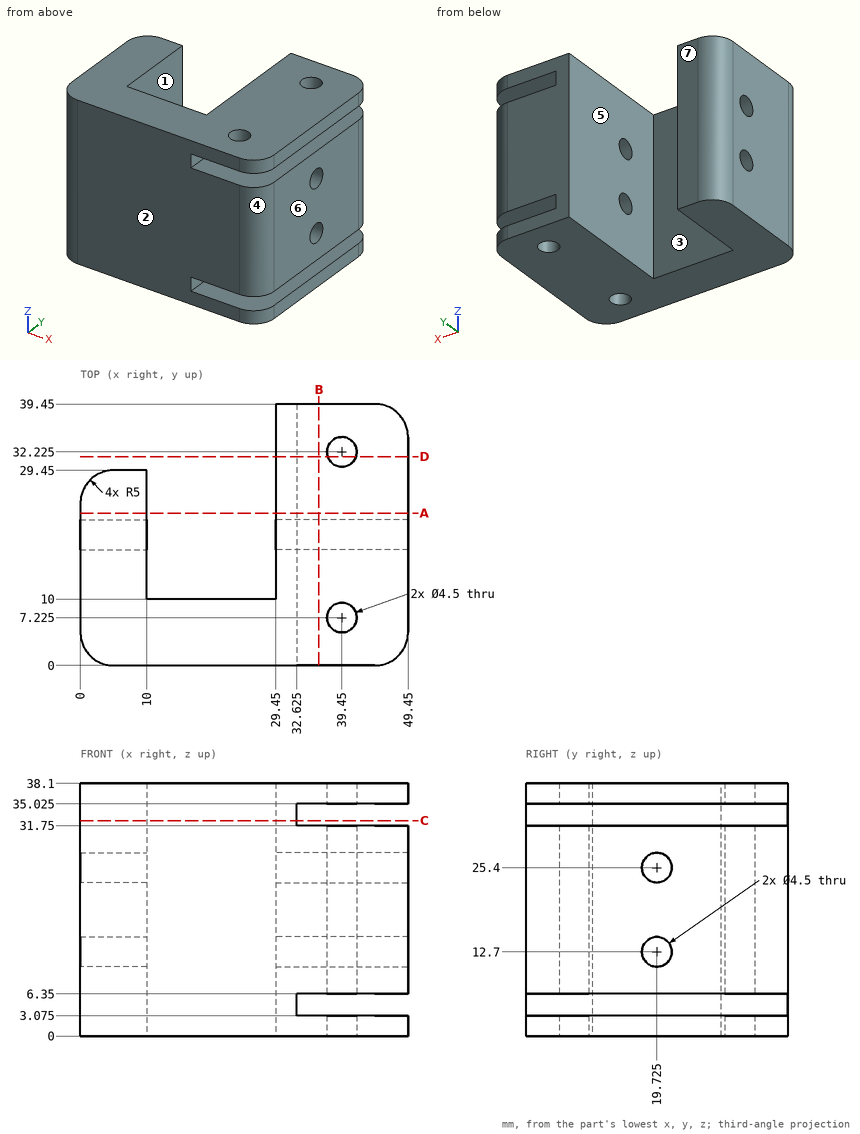
Geometry: see drawing. Coordinates: mm, zero at the bounding-box minimum. A direction names the side the tool comes from. Give positions to 0.01 mm unless a question says otherwise; leave off trailing zeros. Loops run counter-clockwise (first coordinate to the right, second up) from the corner with the lowest first, then second, coordinate; pieces in that order, holes last. Notation, with made-up numbers: (5, -10.5) - (38, -10.5) arc R9 ccw to (38, 3.5) - close; hole circle Ø10 at (-33.75, 57). An arc over 180 degrees is marked (long way). Use CSV: the item, a comma, the result in double quotes. Start each with the question number.
Item 1: Mould query, pull axis X, two halves, no side actions, for the marked faces 1, 2, 3 and 4. Classes: pulls with the +X half, pulls with the -X half, needs draft (parallel to the pull), parting line crosses it, or undercut.
Item 2: Section A-A on y = 23. Return loops of the section in (x, z) (3 decimals), then the cut area to 3 significant figures.
Item 3: Line query: line 1 (Y direction, x = 39.45, z = 36.7) (3 decimals); line 2 (Z direction, x = 45.5, y = 12) (3 decimals); line 3 (Y direction, x = 40.75, z = 12.7) (3 decimals). Output: solid intervals per line, ascending.
Item 4: Reachability of the marked faces 5, 6 and 7 from +Z, -Z, +X, -X, +Y, -Y: full face, straight path, thin tool, end or side. Return the list, or none.
Item 5: Section B-B on x = 36. Return loops of the section in (y, z) (3 decimals), then the cut area to 3 significant figures.
Item 6: Section D-D on y = 31.5. Return loops of the section in (x, z) (3 decimals).
Item 7: Section C-C on z = 32.5. Return loops of the section in (x, y) (3 decimals), then the cut area to 3 significant figures.
Item 8: Contact query for flat-ended pins moving along their axis: P1, Ø3, axis at x = 20, y = 12, coming from the -Z side; P2, Ø6, axis at x = 39.45, y = 32.225, coming from the +Z side; P3, Ø21.5, axis at x = 16, z = 12.5, coming from the +Y side. Output: stop coordinate, or through.
Ans:
1,face 1,"undercut"
1,face 2,"needs draft"
1,face 3,"undercut"
1,face 4,"pulls with the +X half"
2,outline,"(0, 0) - (10, 0) - (10, 38.1) - (0, 38.1) - close; (29.45, 0) - (49.45, 0) - (49.45, 3.075) - (32.625, 3.075) - (32.625, 6.35) - (49.45, 6.35) - (49.45, 31.75) - (32.625, 31.75) - (32.625, 35.025) - (49.45, 35.025) - (49.45, 38.1) - (29.45, 38.1) - close"
2,area,"1,030 mm2"
3,line 1,"y = 0 to 4.975, 9.475 to 29.975, 34.475 to 39.45"
3,line 2,"z = 0 to 3.075, 6.35 to 31.75, 35.025 to 38.1"
3,line 3,"y = 0 to 5.389, 9.061 to 17.475, 21.975 to 30.389, 34.061 to 39.45"
4,face 5,"+Z, -Z, +Y"
4,face 6,"+Z, -Z, +X, +Y, -Y"
4,face 7,"+Z, -Z, -X, +Y"
5,outline,"(0, 0) - (39.45, 0) - (39.45, 3.075) - (0, 3.075) - close; (0, 6.35) - (39.45, 6.35) - (39.45, 31.75) - (0, 31.75) - close; (0, 35.025) - (39.45, 35.025) - (39.45, 38.1) - (0, 38.1) - close; hole circle Ø4.5 at (19.725, 12.7); hole circle Ø4.5 at (19.725, 25.4)"
5,area,"1,210 mm2"
6,outline,"(29.45, 0) - (37.32, 0) - (37.32, 3.075) - (32.625, 3.075) - (32.625, 6.35) - (37.32, 6.35) - (37.32, 31.75) - (32.625, 31.75) - (32.625, 35.025) - (37.32, 35.025) - (37.32, 38.1) - (29.45, 38.1) - close; (41.58, 0) - (49.45, 0) - (49.45, 3.075) - (41.58, 3.075) - close; (41.58, 6.35) - (49.45, 6.35) - (49.45, 31.75) - (41.58, 31.75) - close; (41.58, 35.025) - (49.45, 35.025) - (49.45, 38.1) - (41.58, 38.1) - close"
7,outline,"(0, 5) arc R5 ccw to (5, 0) - (32.625, 0) - (32.625, 39.45) - (29.45, 39.45) - (29.45, 10) - (10, 10) - (10, 29.45) - (5, 29.45) arc R5 ccw to (0, 24.45) - close"
7,area,"604 mm2"
8,P1,"passes through"
8,P2,"stops at z = 38.1"
8,P3,"stops at y = 29.45"
